Geometry check sheet. Reference: the model listing, model coordinates, mm. Face numbers are marked on the shaded views. A direction names the side the tool comes from. Round coordinates to 2 decimals unless told otherwise and drop trailing zeros. Order: outer loops, then holes, each group sorted by start corner. A loop starts at its lowest first (then second) coordinate and runs counter-clockwise, first axis right, second up. Notation, with made-up numbers: (25, 64.5) -> (79, 64.5) arc R27 cw to (79, 102.5) -> close; hole circle Ø8 at (56.5, 50.5). An arc over 180 degrees is marked (long way). Use a Markdown table: item, result. Add a question column.
Item 1: Sectioned sample at A-A, the plane z = 0. Record the cut outline in (x, y), and give its area (3 significant figures).
Item 2: Gauge pin test, flat ends, axial feed: pin 1 Ø1.5 at (y, z) = (-4, -3.5) entering from +X; pin 2 Ø3 at (y, z) = (-3.5, 2) entering from +X; pin 3 Ø1.5 at (x, z) = (3.5, 2.5) entering from -Y. Record the tip position at first contact, or that the pin passes through.
Item 3: Set-up check for the marked faces 1 and 2: record each of +Z, -Z, +X, -X, +Y, -Y from which the full face is reachable in a straight line by a thin tool's end or side.
Item 4: Mould release check, pull along Z, two halves, no side actions. Record for the marked faces 3, 4 and 5: pulls with the +Z half, pulls with the -Z half, needs draft (parallel to the pull), parting line crosses it, or undercut.
Item 5: Material ranges on probe 1 along Y at (x, z) = (2.4, 0); probe 2 along X at (y, z) = (-3, 3.75); probe 3 along Y at (x, z) = (3, 1.75), recorded low to high. Write a range as [from, to].
Item 6: Sectioned sample at D-D, the plane x = 4.5. Record the cut outline in (y, z).
Item 7: Sectioned sample at B-B, the plane x = 2. Record the cut outline in (y, z).
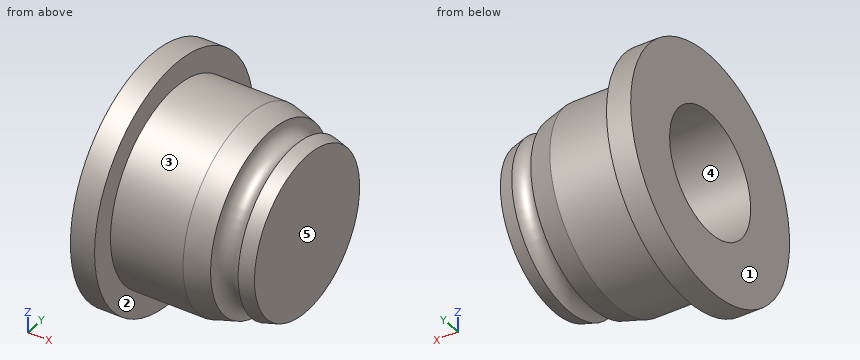
from build123d import *

# Parameters (mm, degrees)
SKETCH3_R               = 1.75
BOSS_EXTRUDE1_DEPTH     = 4
CUT_EXTRUDE1_DEPTH      = 10.604686356
CUT_EXTRUDE1_DEPTH_BACK = 5
SKETCH4_R               = 2.55


with BuildPart() as part:
    # Sketch2 → Revolve1 (revolve)
    with BuildSketch(Plane(origin=(0, 0, 0), x_dir=(1, 0, 0), z_dir=(0, 1, 0)), mode=Mode.PRIVATE) as revolve1_sk:
        with BuildLine():
            Line((0, 0), (0, 5))
            Line((0, 5), (1, 5))
            Line((1, 5), (1, 4))
            Line((1, 4), (4, 4))
            Line((4, 4), (4.962239732, 3.733469404))
            ThreePointArc((4.962239732, 3.733469404), (5.310627067, 3.11814326), (5.925953212, 3.466530596))
            Line((5.925953212, 3.466530596), (6.5, 3.307525488))
            Line((6.5, 3.307525488), (6.5, 0))
            Line((6.5, 0), (0, 0))
        make_face()
    revolve(revolve1_sk.sketch.rotate(Axis((0, 0, 0), (1, 0, 0)), 180), axis=Axis((0, 0, 0), (1, 0, 0)))

    # Sketch3 → Boss-Extrude1 (add)
    with BuildSketch(Plane.ZY):
        Circle(SKETCH3_R)
    extrude(amount=-BOSS_EXTRUDE1_DEPTH)

    # Sketch4 → Cut-Extrude1 (cut, two sides: drawn at the far end of the back side and taken through both)
    with BuildSketch(Plane.ZY.offset(-CUT_EXTRUDE1_DEPTH_BACK)):
        with Locations(Location((0, 0, 0), (0, 0, 180))):
            Circle(SKETCH4_R)
    extrude(amount=CUT_EXTRUDE1_DEPTH + CUT_EXTRUDE1_DEPTH_BACK, mode=Mode.SUBTRACT)


solid = part.part
Found:
| question | item | result |
|---|---|---|
| 1 | outline | (0, -5) -> (1, -5) -> (1, -4) -> (4, -4) -> (4.96, -3.73) arc R0.5 cw to (5.93, -3.47) -> (6.5, -3.31) -> (6.5, 3.31) -> (5.93, 3.47) arc R0.5 cw to (4.96, 3.73) -> (4, 4) -> (1, 4) -> (1, 5) -> (0, 5) -> (0, 2.55) -> (5, 2.55) -> (5, -2.55) -> (0, -2.55) -> close |
| 1 | area | 26.0 mm2 |
| 2 | pin 1 | stops at x = 1 |
| 2 | pin 2 | stops at x = 6.5 |
| 2 | pin 3 | stops at y = -3.6 |
| 3 | face 1 | +Z, -Z, -X, +Y, -Y |
| 3 | face 2 | +X |
| 4 | face 3 | parting line crosses it |
| 4 | face 4 | undercut |
| 4 | face 5 | needs draft |
| 5 | probe 1 | y = [-4, -2.55], [2.55, 4] |
| 5 | probe 2 | x = [0, 1] |
| 5 | probe 3 | y = [-3.6, -1.85], [1.85, 3.6] |
| 6 | outline | circle Ø7.72 at (0, 0); hole circle Ø5.1 at (0, 0) |
| 7 | outline | circle Ø8 at (0, 0); hole circle Ø5.1 at (0, 0) |
